Autodesk Inventor part; units mm, degrees
ref_plane "YZ Plane" through (0, 0, 0) normal (1, 0, 0) x (0, 1, 0)
ref_plane "XZ Plane" through (0, 0, 0) normal (0, 1, 0) x (-1, 0, 0)
ref_plane "XY Plane" through (0, 0, 0) normal (0, 0, 1) x (1, 0, 0)
sketch "スケッチ1" plane through (0, 0, 0) normal (1, 0, 0) x (0, 1, 0)
  line L0 (0, 0) -> (15, 0)
  line L1 (15, 0) -> (15, -15)
  line L2 (15, -15) -> (0, -15)
  line L3 (0, -15) -> (0, 0)
  line L4 (14, -14) -> (14, -1)
  line L5 (14, -1) -> (1, -1)
  line L6 (1, -1) -> (1, -14)
  line L7 (1, -14) -> (14, -14)
  dimension "d0" = 15
  dimension "d1" = 15
  dimension "d2" = 1
extrude "押し出し1" add sketch "スケッチ1" along normal blind 36
sketch "スケッチ2" plane through (0, 0, 0) normal (0, 0, 1) x (1, 0, 0)
  line L0 (0, 15) -> (0, 0)
  line L1 (0, 0) -> (36, 0)
  point P0 (5, 7.5)
  point P1 (25, 7.5)
  dimension "d5" = 5
  dimension "d6" = 20
  dimension "d7" = 7.5
  dimension "d8" = 7.5
sketch "スケッチ3" plane through (0, 15, 0) normal (0, 1, 0) x (1, 0, 0)
  line L0 (0, 15) -> (0, 0)
  line L1 (0, 0) -> (36, 0)
  point P0 (15, 7.5)
  point P1 (30, 7.5)
  dimension "d9" = 15
  dimension "d10" = 15
  dimension "d11" = 7.5
  dimension "d12" = 7.5
hole "穴1" at (5, 7.5, 0) at (25, 7.5, 0) direction (0, 0, -1) diameter 3 end through all
hole "穴2" at (15, 15, -7.5) at (30, 15, -7.5) direction (0, -1, 0) diameter 3 end through all
properties part number "hand-grab-v2-ASP-arm-F-1" material "アルミニウム 6061"
For this review, take the finished solid that the model builds, in its own axes (mm). A direction names the side the tool comes from. Round coordinates to 2 decimals unless told otherwise and drop trailing zeros. Write each loop counter-clockwise with the first axis right and the second up, starting at its lowest first coordinate (ties: lowest second). Pieces come first, ordered by that corner, then holes. Notation, with made-up numbers: (66.5, 62) -> (119.5, 62) arc R30 cw to (119.5, 87) -> close; hole circle Ø4 at (50, 42). An arc over 180 degrees is marked (long way). One line per question, with ' | ' between items. Start each with the question number.
1) Machinability: for faces 1 (the flat face through (18, 8, -15)), 2 (the flat face through (18, 14, -8)), which of the approach directions +Z, -Z, +X, -X, +Y, -Y give a long, thin tool a straight path to every point of the face, cutting with its end or side? Answer none if there is none.
2) Wall thickness on line 1 along X through (y, z) = (7.5, -0.3); line 2 along X through (y, z) = (0.75, -7.5); line 3 along Z through (x, y) = (10, 4.25): over which ranges is each line inside the solid? List them lowest first.
3) Add section A-A (z = -10.25). Write out the cut boundary in (x, y), and give its area (3 significant figures).
4) Mouldability with a two-part tool opening along Y and no side actions: class faces 3 (the cylindrical face through (23.513, 7.695, -0.507)), 4 (the flat face through (18, 7, 0)), 5 (the flat face through (18, 0, -8)) as +Y half, -Y half, draft (parallel to the pull), parting line (faces both ways), or undercut.
5) Add section D-D (y = 7.5). Write out the cut boundary in (x, z).
6) Add section C-C (y = 5.25). Write out the cut boundary in (x, z), and give its area (3 significant figures).
7) Add section B-B (x = 30). Write out the cut boundary in (y, z).
Reported:
1) face 1: -Z, +X, -X, +Y, -Y | face 2: +X, -X
2) line 1: x = 0 to 3.5, 6.5 to 23.5, 26.5 to 36 | line 2: x = 0 to 13.5, 16.5 to 28.5, 31.5 to 36 | line 3: z = -15 to -14, -1 to 0
3) outline: (0, 0) -> (36, 0) -> (36, 1) -> (0, 1) -> close; (0, 14) -> (36, 14) -> (36, 15) -> (0, 15) -> close | area: 72.0 mm²
4) face 3: undercut | face 4: draft | face 5: -Y half
5) outline: (0, -15) -> (3.5, -15) -> (3.5, -14) -> (0, -14) -> close; (0, -1) -> (3.5, -1) -> (3.5, 0) -> (0, 0) -> close; (6.5, -15) -> (23.5, -15) -> (23.5, -14) -> (6.5, -14) -> close; (6.5, -1) -> (23.5, -1) -> (23.5, 0) -> (6.5, 0) -> close; (26.5, -15) -> (36, -15) -> (36, -14) -> (26.5, -14) -> close; (26.5, -1) -> (36, -1) -> (36, 0) -> (26.5, 0) -> close
6) outline: (0, -15) -> (36, -15) -> (36, -14) -> (0, -14) -> close; (0, -1) -> (36, -1) -> (36, 0) -> (0, 0) -> close | area: 72.0 mm²
7) outline: (0, -15) -> (15, -15) -> (15, -9) -> (14, -9) -> (14, -14) -> (1, -14) -> (1, -9) -> (0, -9) -> close; (0, -6) -> (1, -6) -> (1, -1) -> (14, -1) -> (14, -6) -> (15, -6) -> (15, 0) -> (0, 0) -> close
